Design review of the part built by this model. Coordinates are the model's own, in mm. Face numbers are marked on the shaded views. A direction names the side the tool comes from. Coordinates: 2 decimals unless noted, no trailing zeros. Write each loop counter-clockwise with the first axis right and the second up, starting at its lowest first coordinate (ties: lowest second). Pieces come first, ordered by that corner, then holes. Notation, with made-up numbers: M 7,-20.75 L 21,-20.75 A21 cw 21,9.25 Z; hole C -15.5,-8.75 d10. An arc over 180 degrees is marked long. Write item = value, one per line.
```python
from build123d import *

# Parameters (mm, degrees)
SKETCH1_W           = 127
SKETCH1_H           = 50.8
BOSS_EXTRUDE1_DEPTH = 12.7
SHELL1_T            = -1.5875
SKETCH2_R           = 2.4892
CUT_EXTRUDE1_DEPTH  = 140.121529606
SKETCH3_R           = 2.4892
CUT_EXTRUDE2_DEPTH  = 138.371503595
LPATTERN1_COUNT     = 9
LPATTERN1_PITCH     = 12.7


with BuildPart() as part:
    # Sketch1 → Boss-Extrude1 (new, symmetric)
    with BuildSketch(Plane.XY):
        with Locations((63.5, 25.4)):
            Rectangle(SKETCH1_W, SKETCH1_H)
    extrude(amount=BOSS_EXTRUDE1_DEPTH, both=True)

    # Shell1
    shell1_openings = [part.faces().sort_by_distance(p)[0] for p in [
        (127, 25.4, 0),
        (0, 25.4, 0),
    ]]
    offset(amount=SHELL1_T, openings=shell1_openings, kind=Kind.INTERSECTION)

    # Sketch2 → Cut-Extrude1 (cut, through all)
    with BuildSketch(Plane(origin=(0, 0, -12.7), x_dir=(-1, 0, 0), z_dir=(0, 0, -1))):
        with Locations((-114.3, 38.1)):
            Circle(SKETCH2_R)
        with Locations((-114.3, 25.4)):
            Circle(SKETCH2_R)
        with Locations((-114.3, 12.7)):
            Circle(SKETCH2_R)
    cut_extrude1 = extrude(amount=-CUT_EXTRUDE1_DEPTH, mode=Mode.SUBTRACT)

    # Sketch3 → Cut-Extrude2 (cut, through all)
    with BuildSketch(Plane(origin=(0, 50.8, 0), x_dir=(1, 0, 0), z_dir=(0, 1, 0))):
        with Locations(Location((114.3, 0, 0), (0, 0, 270))):
            Circle(SKETCH3_R)
    cut_extrude2 = extrude(amount=-CUT_EXTRUDE2_DEPTH, mode=Mode.SUBTRACT)

    # LPattern1: Cut-Extrude1, Cut-Extrude2 ×9
    with Locations(*[(-i * LPATTERN1_PITCH, 0, 0) for i in range(1, LPATTERN1_COUNT)]):
        add(cut_extrude1, mode=Mode.SUBTRACT)
        add(cut_extrude2, mode=Mode.SUBTRACT)


solid = part.part
```
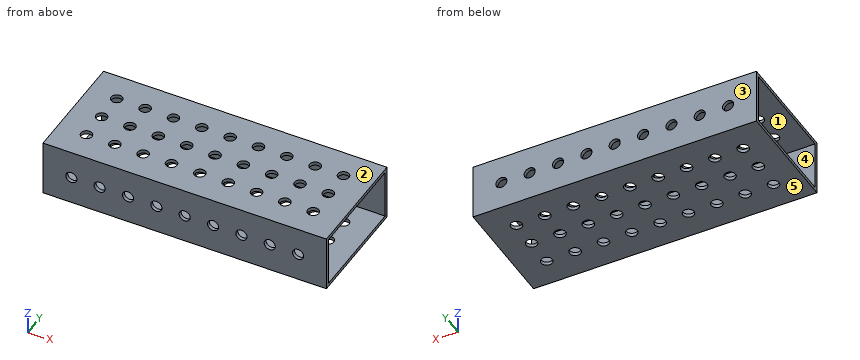
Q1. For P1, Ø3, axis at x = 101.6, y = 25.4, coming from the +Z side, flat-tipped, find the tip position at first contact; note if it passes through.
Check result:
P1 = through
Q2. Machinability: for the marked faces 4 and 5, which of the approach directions +Z, -Z, +X, -X, +Y, -Y give a long, thin tool a straight path to every point of the face, cutting with its end or side? Answer none if there is none.
Check result:
face_4 = +X, -X
face_5 = -Z, +X, -X, +Y, -Y
Q3. Consider section B-B, the plane z = 9. State the section outline as (x, y) points, and give its area (3 significant figures).
Check result:
outline = M 0,0 L 127,0 L 127,1.59 L 0,1.59 Z; M 0,49.21 L 127,49.21 L 127,50.8 L 0,50.8 Z
area = 403 mm²
Q4. Consider section A-A, the plane x = 83. State the section outline as (y, z) points, and give its area (3 significant figures).
Check result:
outline = M 0,-12.7 L 50.8,-12.7 L 50.8,12.7 L 0,12.7 Z; hole M 1.59,-11.11 L 49.21,-11.11 L 49.21,11.11 L 1.59,11.11 Z
area = 232 mm²
Q5. Wall thickness on line 1 (Y direction, x = 114.3, z = -11.75); line 2 (Z direction, x = 98, y = 22); line 3 (Y direction, x = 121, z = -9.75): over which ranges is each line inside the solid? List them lowest first.
Check result:
line_1 = 0 to 10.21, 15.19 to 22.91, 27.89 to 35.61, 40.59 to 50.8
line_2 = -12.7 to -11.11, 11.11 to 12.7
line_3 = 0 to 1.59, 49.21 to 50.8
Q6. The part is to be moulded in two halves that separate along Z. For the marked faces 1, 2 and 3, say which applies: +Z half, -Z half, draft (parallel to the pull), parting line (faces both ways), or undercut.
Check result:
face_1 = undercut
face_2 = +Z half
face_3 = draft
Q7. Consider section C-C, the plane y = 21. State the section outline as (x, z) points.
Check result:
outline = M 0,-12.7 L 127,-12.7 L 127,-11.11 L 0,-11.11 Z; M 0,11.11 L 127,11.11 L 127,12.7 L 0,12.7 Z
Q8. Consider section D-D, the plane x = 25.4. State how many separate pieces and enclosed holes the cut face has, and give its area (3 significant figures).
Check result:
separate_pieces = 8
enclosed_holes = 0
area = 169 mm²
